Geometry: see drawing. Coordinates: mm, zero at the bounding-box minimum. Round coordinates to 2 decimals unless told otherwise and drop trailing zeros. Write each loop counter-clockwise with the first axis right and the second up, starting at its lowest first coordinate (ties: lowest second). Pieces come first, ordered by that corner, then holes. Notation, with made-up numbers: (12, 37.5) -> (18, 37.5) arc R17 cw to (18, 47.5) -> close; hole circle Ø7 at (59.5, 23). An arc over 180 degrees is marked (long way). Use CSV: the item, a comma, the result in double quotes.
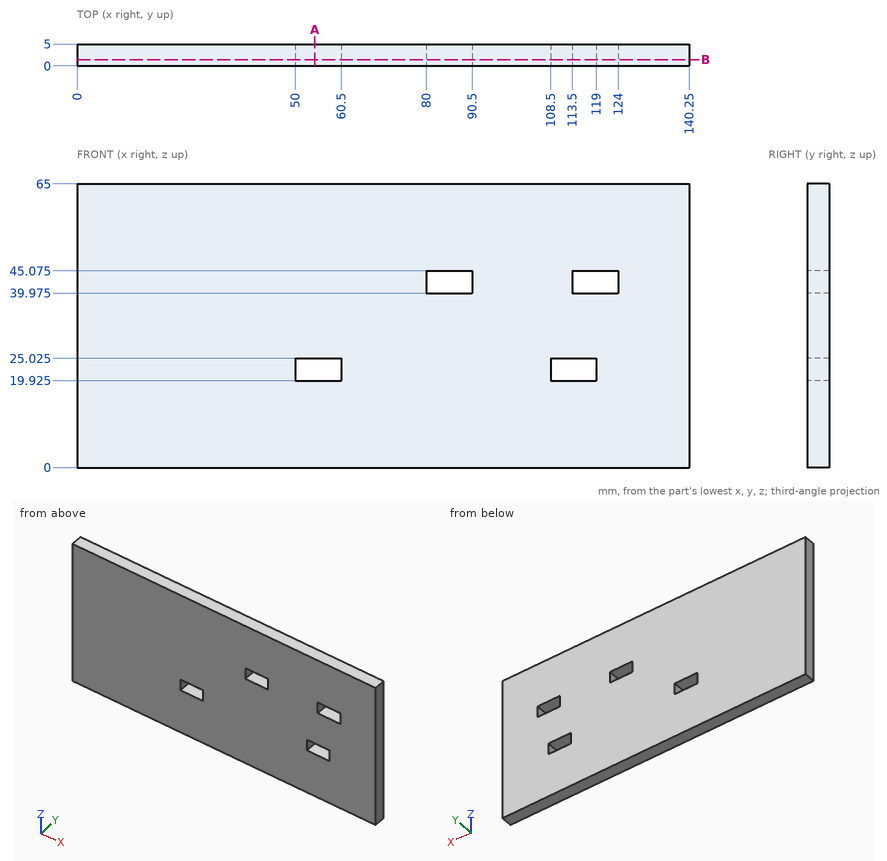
Item 1: Section query B-B on y = 1.4. Return the cut outline in (x, z) (3 decimals), plus the area to 3 significant figures.
Worked answers:
outline,"(0, 0) -> (140.25, 0) -> (140.25, 65) -> (0, 65) -> close; hole (50, 19.925) -> (60.5, 19.925) -> (60.5, 25.025) -> (50, 25.025) -> close; hole (80, 39.975) -> (90.5, 39.975) -> (90.5, 45.075) -> (80, 45.075) -> close; hole (108.5, 19.925) -> (119, 19.925) -> (119, 25.025) -> (108.5, 25.025) -> close; hole (113.5, 39.975) -> (124, 39.975) -> (124, 45.075) -> (113.5, 45.075) -> close"
area,"8,900 mm²"
Item 2: Section query A-A on x = 54.5. Return the cut outline in (y, z) (3 decimals), plus the area to 4 significant figures.
Worked answers:
outline,"(0, 0) -> (5, 0) -> (5, 19.925) -> (0, 19.925) -> close; (0, 25.025) -> (5, 25.025) -> (5, 65) -> (0, 65) -> close"
area,"299.5 mm²"
Item 3: Line query: line 1 (X direction, y = 3.15, z = 22); line 2 (Z direction, x = 118.5, y = 1.35) (3 decimals); line 3 (X direction, y = 4, z = 44). Output: solid intervals per line, ascending.
Worked answers:
line 1,"x = 0 to 50, 60.5 to 108.5, 119 to 140.25"
line 2,"z = 0 to 19.925, 25.025 to 39.975, 45.075 to 65"
line 3,"x = 0 to 80, 90.5 to 113.5, 124 to 140.25"
